Geometry check sheet. Reference: the model listing, model coordinates, mm. A direction names the side the tool comes from. Give positions to 0.01 mm unless a question says otherwise; leave off trailing zeros. Loops run counter-clockwise (first coordinate to the right, second up) from the corner with the lowest first, then second, coordinate; pieces in that order, holes last. Notation, with made-up numbers: (67, 77) - (85, 77) arc R23 ccw to (85, 103) - close; hole circle Ø6 at (-33, -24). An arc over 180 degrees is marked (long way). Use a Markdown table: item, result. Add a question column.
1. Draft check along Z on faces 4 (the cylindrical face through (0.133, -82.531, -63.282)), 5 (the flat face through (12.5, -47, -58)), 6 (the cylindrical face through (-3.58, 17.34, -78.1)). Enter one of: pulls with the +Z half, pulls with the -Z half, needs draft (parallel to the pull), parting line crosses it, or undercut.
2. Material ranges on L1, parallel to Z at x = 5.75, y = 0; L2, parallel to Z at x = -1.5, y = 0; L3, parallel to Y at x = -4, z = 5.5, recorded low to high.
3. Cross-section at A-A on z = 0. Enter the section's corners in (x, y).
4. Cross-section at B-B on x = -2.5. Enter the section's corners in (y, z).
5. Depth check by flat-ended pin: P1, Ø8.5, axis at y = -93, z = 0, coming from the -X side; P2, Ø6, axis at x = 7.5, y = 12.5, coming from the -Z side; P3, Ø8, axis at y = -76.5, z = 47, coming from the +X side; P4, Ø2, axis at x = 2, z = -14.5, coming from the -Y side. Enter the tip coordinate at first touch or a pass-through.
6. Cross-section at C-C on y = -93. Enter the section's corners in (x, z), and give its area (3 significant figures).
7. Set-up check for faces 1 (the cylindrical face through (10.49, -17.34, -78.1)), 2 (the flat face through (2.5, -59, 36)), 3 (the cylindrical face through (-0.13, 0.91, -86.06)): record each of +Z, -Z, +X, -X, +Y, -Y from which the full face is reachable in a straight line by a thin tool's end or side.
from build123d import *

# Parameters (mm, degrees)
F0_R     = 104
F0_R_2   = 68.5
F1_DEPTH = 9.5
F3_D     = 14
F4_R     = 80
F5_DEPTH = 12
F6_R     = 80
F6_R_2   = 68.5
F7_DEPTH = 3
F8_SIZE  = 1
F9_SIZE  = 6


with BuildPart() as f1:
    # F0 (on Right) → F1 (new body, symmetric)
    with BuildSketch(Plane.YZ):
        Circle(F0_R)
        Circle(F0_R_2, mode=Mode.SUBTRACT)
    extrude(amount=F1_DEPTH, both=True)

    # F3 (through all)
    with Locations(Plane.YZ.offset(9.5)):
        with Locations((0, 93), (93, 0), (0, -93), (-93, 0)):
            Hole(F3_D / 2)

    # F4 (on face) → F5 (cut)
    with BuildSketch(Plane(origin=(-9.5, 0, 0), x_dir=(0, -1, 0), z_dir=(-1, 0, 0))):
        Circle(F4_R)
    extrude(amount=-F5_DEPTH, mode=Mode.SUBTRACT)

    # F6 (on face) → F7 (join)
    with BuildSketch(Plane.YZ.offset(9.5)):
        Circle(F6_R)
        Circle(F6_R_2, mode=Mode.SUBTRACT)
    extrude(amount=F7_DEPTH)

    # F8
    f8_edges = [f1.edges().sort_by_distance(p)[0] for p in [
        (12.5, -80, 0),
    ]]
    chamfer(f8_edges, length=F8_SIZE)

    # F9
    f9_edges = [f1.edges().sort_by_distance(p)[0] for p in [
        (12.5, -68.5, 0),
    ]]
    chamfer(f9_edges, length=F9_SIZE)


solid = f1.part
Values found:
| question | item | result |
|---|---|---|
| 1 | face 4 | parting line crosses it |
| 1 | face 5 | needs draft |
| 1 | face 6 | undercut |
| 2 | L1 | z = -104 to -100, -86 to -68.5, 68.5 to 86, 100 to 104 |
| 2 | L2 | z = -104 to -100, -86 to -80, 80 to 86, 100 to 104 |
| 2 | L3 | y = -103.85 to -97.33, -88.67 to -79.81, 79.81 to 88.67, 97.33 to 103.85 |
| 3 | outline | (-9.5, -104) - (9.5, -104) - (9.5, -100) - (-9.5, -100) - close; (-9.5, -86) - (9.5, -86) - (9.5, -80) - (11.5, -80) - (12.5, -79) - (12.5, -74.5) - (6.5, -68.5) - (2.5, -68.5) - (2.5, -80) - (-9.5, -80) - close; (-9.5, 80) - (2.5, 80) - (2.5, 68.5) - (6.5, 68.5) - (12.5, 74.5) - (12.5, 79) - (11.5, 80) - (9.5, 80) - (9.5, 86) - (-9.5, 86) - close; (-9.5, 100) - (9.5, 100) - (9.5, 104) - (-9.5, 104) - close |
| 4 | outline | circle Ø208 at (0, 0); hole circle Ø14 at (-93, 0); hole circle Ø160 at (0, 0); hole circle Ø14 at (0, -93); hole circle Ø14 at (0, 93); hole circle Ø14 at (93, 0) |
| 5 | P1 | passes through |
| 5 | P2 | stops at z = -103.57 |
| 5 | P3 | stops at x = 9.5 |
| 5 | P4 | stops at y = -103.12 |
| 6 | outline | (-9.5, -46.55) - (9.5, -46.55) - (9.5, -7) - (-9.5, -7) - close; (-9.5, 7) - (9.5, 7) - (9.5, 46.55) - (-9.5, 46.55) - close |
| 6 | area | 1,500 mm2 |
| 7 | face 1 | +X |
| 7 | face 2 | -X |
| 7 | face 3 | +X, -X |
